Verification items for the finished model (mm, model axes). Face numbers are marked on the shaded views. Round coordinates to 2 decimals unless told otherwise and drop trailing zeros. Write each loop counter-clockwise with the first axis right and the second up, starting at its lowest first coordinate (ties: lowest second). Pieces come first, ordered by that corner, then holes. Notation, with made-up numbers: M 6,-13 L 63,-13 A11 cw 63,8 Z; hole C 34.5,-31 d6. An arc over 180 degrees is marked long. One line per question, with ' | ' between items. Start each with the question number.
Q1. Release check for a two-part mould opening along X. For the marked faces 1, 2 and 3 record: released by +X, released by -X, zero draft, split by the parting line, or undercut.
Q2. Cross-section at A-A (y = 0). Record the boundary of the cut face in (x, z) (1 decimal).
Q3. Thickness scan on line 1 along Y through (x, z) = (0, 0.95) (1 decimal); line 2 along X through (y, z) = (1.5, 0.8); line 3 along Y through (x, z) = (-2, 0.3). Record the ranges inside material, lowest first. Write a range as from..to.
Q4. Gauge pin test, flat ends, axial feed: pin 1 (3 mm diameter, centred on x = 3.5, y = 2.5, fed in from -Z); pin 2 (1 mm diameter, centred on x = 4.5, z = 0.5, fed in from +Y). Record the tip position at first contact, or that the pin passes through.
Q5. Cross-section at D-D (x = -4.25). Record the boundary of the cut face in (y, z).
Autodesk Inventor part; units mm, degrees
ref_plane "YZ Plane" through (0, 0, 0) normal (1, 0, 0) x (0, 1, 0)
ref_plane "XZ Plane" through (0, 0, 0) normal (0, 1, 0) x (-1, 0, 0)
ref_plane "XY Plane" through (0, 0, 0) normal (0, 0, 1) x (1, 0, 0)
sketch "Sketch1" plane through (0, 0, 0) normal (0, 0, 1) x (1, 0, 0)
  circle A0 centre (0, 0) radius 7.9375
  circle A1 centre (0, 0) radius 3.175
  dimension "d0" = 15.875
  dimension "d1" = 6.35
extrude "Extrusion1" add sketch "Sketch1" along normal blind 2.032
sketch "Sketch2" plane through (0, 0, 2.032) normal (0, 0, 1) x (1, 0, 0)
  circle A0 centre (0, 0) radius 7.9375 construction
  arc A1 (2.0793, 5.1162) -> (0.2784, 17.7544) centre (-62.2212, 2.4011) ccw
  arc A2 (14.1052, 14.1744) -> (6.3972, 3.9982) centre (61.3005, -29.5808) ccw
  arc A3 (6.3972, 3.9982) -> (2.0793, 5.1162) centre (-39.8868, -165.864) ccw
  arc A4 (6.6263, 4.3699) -> (1.9179, 7.7023) centre (0, 0) ccw
extrude "Extrusion2" cut sketch "Sketch2" against normal blind 25.4
properties part number "Gear Washer Spacer 3" material "Steel"
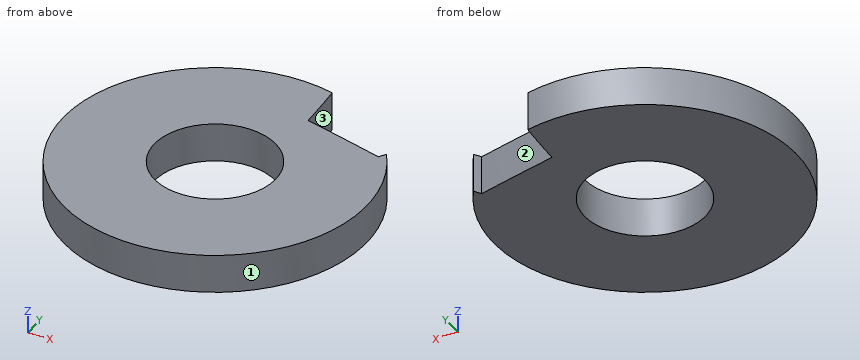
Determined:
1) face 1: split by the parting line | face 2: undercut | face 3: released by +X
2) outline: M -7.9,0 L -3.2,0 L -3.2,2 L -7.9,2 Z; M 3.2,0 L 7.9,0 L 7.9,2 L 3.2,2 Z
3) line 1: y = -7.9..-3.2, 3.2..7.9 | line 2: x = -7.79..-2.8, 2.8..7.79 | line 3: y = -7.68..-2.47, 2.47..7.68
4) pin 1: stops at z = 0 | pin 2: stops at y = 4.63
5) outline: M -6.7,0 L 6.7,0 L 6.7,2.03 L -6.7,2.03 Z
